Check sheet for the modelled part. Datum: model origin and axes. Units: mm. A direction names the side the tool comes from. Round coordinates to 2 decimals unless told otherwise and drop trailing zeros. Order: outer loops, then holes, each group sorted by start corner. A loop starts at its lowest first (then second) coordinate and runs counter-clockwise, first axis right, second up.
Q1. Cross-section at C-C on y = 3. Record the cut outline in (x, z), then the cut area to 3 significant figures.
Q2. Mould release check, pull along Z, two halves, no side actions. Record for faces 4 (the cylindrical face through (9.59, 2.46, -18.43)), 5 (the cylindrical face through (-15.37, 2.46, 11.4)), 6 (the flat face through (0, 5, 0)): +Z half, -Z half, draft (parallel to the pull), parting line (faces both ways), or undercut.
Q3. Set-up check for faces 1 (the flat face through (0, -10, 0)), 2 (the flat face through (13.87, 2.46, 10.11)), 3 (the cylindrical face through (-5.158, -4.93, -3.955)): record each of +Z, -Z, +X, -X, +Y, -Y from which the full face is reachable in a straight line by a thin tool's end or side.
Q4. Cross-section at B-B on z = 10.5. Record the cut outline in (x, y), then the cut area to 3 significant figures.
Q5. Cross-section at A-A on x = 0. Record the cut outline in (y, z), then the cut area to 3 significant figures.
Q6. Depth check by flat-ended pin: P1, Ø5, axis at x = 16, y = 1.5, coming from the -Z side; P2, Ø1.5, axis at x = -11, y = 2, coming from the -Z side; P3, Ø2, axis at x = 9, z = 13, coming from the -Y side. Enter the tip coordinate at first touch or a pass-through.
Q7. Cross-section at D-D on z = 0. Record the cut outline in (x, y), then the cut area to 3 significant figures.
Q8. Scan lines: probe 1 along Y at (x, z) = (8, -19); probe 2 along Z at (x, y) = (-1, 2); probe 3 along Z at (x, y) = (-15.5, 1.5). Record each from-to range of solid material in increasing order.
from build123d import *

# Parameters (mm, degrees)
F0_R     = 6.5
F1_DEPTH = 10
F2_R     = 20.7743809462
F3_DEPTH = 5
F5_DEPTH = 25


with BuildPart() as f1:
    # F0 (on Front) → F1 (new body)
    with BuildSketch(Plane.XZ):
        Circle(F0_R)
    extrude(amount=F1_DEPTH)

    # F2 (on Front) → F3 (join)
    with BuildSketch(Plane.XZ):
        Circle(F2_R)
    extrude(amount=-F3_DEPTH)

    # F4 (on face) → F5 (cut)
    with BuildSketch(Plane.XZ):
        with BuildLine():
            Line((-9.9486096802, 11.406318953), (-12.577847041, 14.4208024743))
            ThreePointArc((-12.577847041, 14.4208024743), (-15.4009347645, 11.3566275174), (-17.493895192, 7.7540577249))
            Line((-17.493895192, 7.7540577249), (-13.8370211121, 6.1331715588))
            ThreePointArc((-13.8370211121, 6.1331715588), (-12.1815671778, 8.9826704114), (-9.9486096802, 11.406318953))
        make_face()
        with BuildLine():
            Line((14.8524668171, 2.9125892389), (18.7777048063, 3.6823338253))
            ThreePointArc((18.7777048063, 3.6823338253), (17.5355953137, 7.6592869894), (15.4621585682, 11.273128785))
            Line((15.4621585682, 11.273128785), (12.2299929317, 8.9166260164))
            ThreePointArc((12.2299929317, 8.9166260164), (13.870004359, 6.0582114282), (14.8524668171, 2.9125892389))
        make_face()
        with BuildLine():
            ThreePointArc((-6.1998577652, -18.1031362996), (-2.1346605491, -19.0159145068), (2.0317366238, -19.0271865099))
            Line((2.0317366238, -19.0271865099), (1.6070281804, -15.0497975752))
            ThreePointArc((1.6070281804, -15.0497975752), (-1.6884371812, -15.0408818396), (-4.9038571369, -14.3189081919))
            Line((-4.9038571369, -14.3189081919), (-6.1998577652, -18.1031362996))
        make_face()
    extrude(amount=-F5_DEPTH, mode=Mode.SUBTRACT)


solid = f1.part
Results found:
1. outline: circle Ø41.55 at (0, 0); hole (-17.49, 7.75) - (-13.84, 6.13) arc R15.14 cw to (-9.95, 11.41) - (-12.58, 14.42) arc R19.14 ccw to start; hole (-6.2, -18.1) arc R19.14 ccw to (2.03, -19.03) - (1.61, -15.05) arc R15.14 cw to (-4.9, -14.32) - close; hole (12.23, 8.92) arc R15.14 cw to (14.85, 2.91) - (18.78, 3.68) arc R19.14 ccw to (15.46, 11.27) - close
1. area: 1,270 mm2
2. face 4: parting line
2. face 5: undercut
2. face 6: draft
3. face 1: +Z, -Z, +X, -X, -Y
3. face 2: +Y, -Y
3. face 3: -Y
4. outline: (-17.93, 0) - (-16, 0) - (-16, 5) - (-17.93, 5) - close; (-10.9, 0) - (14.4, 0) - (14.4, 5) - (-10.9, 5) - close; (16, 0) - (17.93, 0) - (17.93, 5) - (16, 5) - close
4. area: 146 mm2
5. outline: (-10, -6.5) - (0, -6.5) - (0, -15.14) - (5, -15.14) - (5, 20.77) - (0, 20.77) - (0, 6.5) - (-10, 6.5) - close; (0, -20.77) - (5, -20.77) - (5, -19.14) - (0, -19.14) - close
5. area: 318 mm2
6. P1: stops at z = -15.79
6. P2: stops at z = -18.07
6. P3: stops at y = 0
7. outline: (-20.77, 0) - (-6.5, 0) - (-6.5, -10) - (6.5, -10) - (6.5, 0) - (20.77, 0) - (20.77, 5) - (-20.77, 5) - close
7. area: 338 mm2
8. probe 1: y = 0 to 5
8. probe 2: z = -20.75 to -19.11, -15.1 to 20.75
8. probe 3: z = -13.83 to 6.87, 11.22 to 13.83
